Geometry check sheet. Reference: the model listing, model coordinates, mm. Face numbers are marked on the shaded views. A direction names the side the tool comes from. Round coordinates to 2 decimals unless told otherwise and drop trailing zeros. Loops run counter-clockwise (first coordinate to the right, second up) from the corner with the lowest first, then second, coordinate; pieces in that order, holes last. Notation, with made-up numbers: (11.25, -2) -> (46.25, -2) arc R35 ccw to (46.25, 30) -> close; hole circle Ø5 at (61, 74). An arc over 180 degrees is marked (long way). Use a Markdown table: item, result. Add a question column.
Q1. Sectioned sample at A-A, the plane y = 2.75. Enter the section's corners in (x, z), then the cut area to 3 significant figures.
Q2. Gauge pin test, flat ends, axial feed: P1, Ø1.6, axis at x = 3.5, y = -10.5, coming from the +Z side; P2, Ø2, axis at x = -5.5, y = -11, coming from the -Z side; P3, Ø7.5, axis at x = 0, y = -1, coming from the +Z side; P4, Ø1, axis at x = 8, y = -3.5, coming from the -Z side. Record the tip position at first contact, or that the pin passes through.
Q3. Sectioned sample at D-D, the plane z = 13. Enter the section's corners in (x, y), then the cut area to 3 significant figures.
Q4. Release check for a two-part mould opening along Y. For the marked faces 1, 2 and 3 record: released by +Y, released by -Y, zero draft, split by the parting line, or undercut.
Q5. Sectioned sample at B-B, the plane z = 8. Enter the section's corners in (x, y).
Q6. Sectioned sample at C-C, the plane x = 0. Enter the section's corners in (y, z).
Q7. Set-up check for the marked faces 4, 5, 6 and 7: record each of +Z, -Z, +X, -X, +Y, -Y from which the full face is reachable in a straight line by a thin tool's end or side.
Q8. Material ranges on L1, parallel to X at y = 0, z = 16.5; L2, parallel to Y at x = 0, z = 7; L3, parallel to Y at x = 5.25, z = 5.5, recorded low to high.
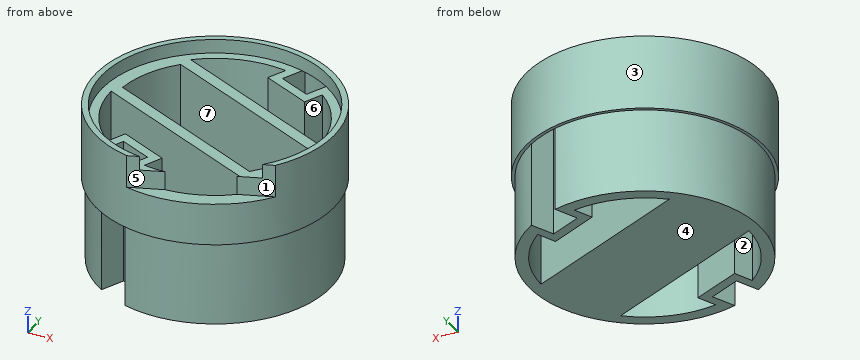
```python
from build123d import *

# Parameters (mm, degrees)
SKETCH_1_R          = 12.4
EXTRUDE_1_DEPTH     = 17
SKETCH_2_R          = 12.1
CUT_EXTRUDE_1_DEPTH = 1.5
CUT_EXTRUDE_2_DEPTH = 24.404486749
EXTRUDE_START       = -8
SKETCH_4_R          = 12.75
SKETCH_4_R_2        = 12.4
EXTRUDE_2_DEPTH     = 8
CUT_EXTRUDE_3_DEPTH = 14.5
CUT_EXTRUDE_4_DEPTH = 24.777615524
CUT_EXTRUDE_START   = -3.5
CUT_EXTRUDE_5_DEPTH = 3.5


with BuildPart() as part:
    # 草图1 → 凸台-拉伸1 (new body)
    with BuildSketch(Plane.XY):
        Circle(SKETCH_1_R)
    extrude(amount=EXTRUDE_1_DEPTH)

    # 草图2 → 切除-拉伸1 (cut)
    with BuildSketch(Plane.XY.offset(17)):
        Circle(SKETCH_2_R)
    extrude(amount=-CUT_EXTRUDE_1_DEPTH, mode=Mode.SUBTRACT)

    # 草图3 → 切除-拉伸2 (cut, through all)
    with BuildSketch(Plane.XY.offset(15.5)):
        with BuildLine():
            Line((-6.915466109, -10.292537515), (-5.774584306, -7.870847726))
            Line((-5.774584306, -7.870847726), (-2.405724389, -9.457950665))
            Line((-2.405724389, -9.457950665), (-3.547574837, -11.881696544))
            ThreePointArc((-3.547574837, -11.881696544), (-5.291518031, -11.214269345), (-6.915466109, -10.292537515))
        make_face()
        with BuildLine():
            Line((5.761046975, 7.877225296), (6.902897424, 10.300971175))
            ThreePointArc((6.902897424, 10.300971175), (5.277825448, 11.220720055), (3.533068862, 11.886018022))
            Line((3.533068862, 11.886018022), (2.392187058, 9.464328234))
            Line((2.392187058, 9.464328234), (5.761046975, 7.877225296))
        make_face()
    extrude(amount=-CUT_EXTRUDE_2_DEPTH, mode=Mode.SUBTRACT)

    # 草图4 → 凸台-拉伸2 (add)
    with BuildSketch(Plane.XY.offset(17).offset(EXTRUDE_START)):
        Circle(SKETCH_4_R)
        Circle(SKETCH_4_R_2, mode=Mode.SUBTRACT)
    extrude(amount=EXTRUDE_2_DEPTH)

    # 草图5 → 切除-拉伸3 (cut)
    with BuildSketch(Plane.XY.offset(15.5)):
        with BuildLine():
            Line((-7.463806301, 7.385228195), (10.44708929, -1.05277033))
            ThreePointArc((10.44708929, -1.05277033), (9.498686797, -4.474924483), (7.463806301, -7.385228195))
            Line((7.463806301, -7.385228195), (-10.44708929, 1.05277033))
            ThreePointArc((-10.44708929, 1.05277033), (-9.498686797, 4.474924483), (-7.463806301, 7.385228195))
        make_face()
    extrude(amount=-CUT_EXTRUDE_3_DEPTH, mode=Mode.SUBTRACT)

    # 草图6 → 切除-拉伸4 (cut, through all)
    with BuildSketch(Plane.XY.offset(15.5)):
        with BuildLine():
            Line((11.09973429, 0.076802961), (-7.008374763, 8.607710682))
            ThreePointArc((-7.008374763, 8.607710682), (-2.770642176, 10.748653029), (1.973996084, 10.923064564))
            Line((1.973996084, 10.923064564), (1.061366936, 8.98587468))
            Line((1.061366936, 8.98587468), (6.239500529, 6.546405174))
            Line((6.239500529, 6.546405174), (7.153831598, 8.487207636))
            ThreePointArc((7.153831598, 8.487207636), (10.048974754, 4.714669277), (11.09973429, 0.076802961))
        make_face()
        with BuildLine():
            Line((7.008374763, -8.607710682), (-11.09973429, -0.076802961))
            ThreePointArc((-11.09973429, -0.076802961), (-10.052261546, -4.707657359), (-7.165667007, -8.477217488))
            Line((-7.165667007, -8.477217488), (-6.253037859, -6.540027604))
            Line((-6.253037859, -6.540027604), (-1.074904267, -8.979497111))
            Line((-1.074904267, -8.979497111), (-1.989235336, -10.920299574))
            ThreePointArc((-1.989235336, -10.920299574), (2.763142593, -10.75058338), (7.008374763, -8.607710682))
        make_face()
    extrude(amount=-CUT_EXTRUDE_4_DEPTH, mode=Mode.SUBTRACT)

    # 草图7 → 切除-拉伸5 (cut)
    with BuildSketch(Plane.XY.offset(17).offset(CUT_EXTRUDE_START)):
        with BuildLine():
            Line((-3.16472158, -12.350993374), (10.31093311, -7.499810558))
            ThreePointArc((10.31093311, -7.499810558), (4.318631553, -11.996329502), (-3.16472158, -12.350993374))
        make_face()
    extrude(amount=CUT_EXTRUDE_5_DEPTH, mode=Mode.SUBTRACT)


solid = part.part
```
Values:
| question | item | result |
|---|---|---|
| 1 | outline | (-12.45, 9) -> (-12.09, 9) -> (-12.09, 0) -> (5.43, 0) -> (5.43, 15.5) -> (2.38, 15.5) -> (2.38, 1) -> (-10.13, 1) -> (-10.13, 15.5) -> (-11.78, 15.5) -> (-11.78, 17) -> (-12.45, 17) -> close; (10.75, 0) -> (12.09, 0) -> (12.09, 9) -> (12.45, 9) -> (12.45, 17) -> (11.78, 17) -> (11.78, 15.5) -> (10.75, 15.5) -> close |
| 1 | area | 118 mm^2 |
| 2 | P1 | z = 13.5 |
| 2 | P2 | z = 9 |
| 2 | P3 | z = 15.5 |
| 2 | P4 | z = 0 |
| 3 | outline | circle Ø25.5 at (0, 0); hole (-11.1, -0.08) arc R11.1 ccw to (-7.17, -8.48) -> (-6.25, -6.54) -> (-1.07, -8.98) -> (-1.99, -10.92) arc R11.1 ccw to (7.01, -8.61) -> close; hole (-10.45, 1.05) -> (7.46, -7.39) arc R10.5 ccw to (10.45, -1.05) -> (-7.46, 7.39) arc R10.5 ccw to start; hole (-7.01, 8.61) -> (11.1, 0.08) arc R11.1 ccw to (7.15, 8.49) -> (6.24, 6.55) -> (1.06, 8.99) -> (1.97, 10.92) arc R11.1 ccw to start; hole (-6.92, -10.29) arc R12.4 ccw to (-3.55, -11.88) -> (-2.41, -9.46) -> (-5.77, -7.87) -> close; hole (2.39, 9.46) -> (5.76, 7.88) -> (6.9, 10.3) arc R12.4 ccw to (3.53, 11.89) -> close |
| 3 | area | 192 mm^2 |
| 4 | face 1 | released by -Y |
| 4 | face 2 | undercut |
| 4 | face 3 | split by the parting line |
| 5 | outline | (-6.92, -10.29) -> (-5.77, -7.87) -> (-2.41, -9.46) -> (-3.55, -11.88) arc R12.4 ccw to (6.9, 10.3) -> (5.76, 7.88) -> (2.39, 9.46) -> (3.53, 11.89) arc R12.4 ccw to start; hole (-11.1, -0.08) arc R11.1 ccw to (-7.17, -8.48) -> (-6.25, -6.54) -> (-1.07, -8.98) -> (-1.99, -10.92) arc R11.1 ccw to (7.01, -8.61) -> close; hole (-10.45, 1.05) -> (7.46, -7.39) arc R10.5 ccw to (10.45, -1.05) -> (-7.46, 7.39) arc R10.5 ccw to start; hole (-7.01, 8.61) -> (11.1, 0.08) arc R11.1 ccw to (7.15, 8.49) -> (6.24, 6.55) -> (1.06, 8.99) -> (1.97, 10.92) arc R11.1 ccw to start |
| 6 | outline | (-12.75, 9) -> (-12.4, 9) -> (-12.4, 0) -> (-11.1, 0) -> (-11.1, 15.5) -> (-11.21, 15.5) -> (-11.21, 13.5) -> (-12.75, 13.5) -> close; (-5.31, 0) -> (5.31, 0) -> (5.31, 15.5) -> (3.87, 15.5) -> (3.87, 1) -> (-3.87, 1) -> (-3.87, 15.5) -> (-5.31, 15.5) -> close; (11.1, 0) -> (12.4, 0) -> (12.4, 9) -> (12.75, 9) -> (12.75, 17) -> (12.1, 17) -> (12.1, 15.5) -> (11.1, 15.5) -> close |
| 7 | face 4 | -Z, +X, -X, +Y, -Y |
| 7 | face 5 | +Z, +X, -Y |
| 7 | face 6 | +Z, -Z |
| 7 | face 7 | +Z |
| 8 | L1 | -12.75 to -12.1, 12.1 to 12.75 |
| 8 | L2 | -12.4 to -11.1, -5.31 to -3.87, 3.87 to 5.31, 11.1 to 12.4 |
| 8 | L3 | -11.23 to -9.78, -7.78 to -6.34, 1.4 to 2.83, 7.01 to 8.12 |
